Print and shaded views of the part. All mm, measured from the part's lowest x, y and z. A direction names the side the tool comes from. Round coordinates to 2 decimals unless told otherwise and drop trailing zeros. Order: outer loops, then holes, each group sorted by start corner. A loop starts at its lowest first (then second) coordinate and runs counter-clockwise, first axis right, second up. Notation, with made-up numbers: (81, 29) - (99, 29) arc R30 cw to (99, 61) - close; hole circle Ø7 at (18.5, 88.25). An arc over 180 degrees is marked (long way). Return JSON: item names as keys, results as strings. Group by question number.
Item 1: Probe probe 1 along X at (y, z) = (39.5, 5.75); probe 2 along Y at (x, z) = (40, 2.15); probe 3 along Z at (x, y) = (44, 29). List the from-to ranges inside material, lowest first.
Item 2: Saw through at A-A on x = 40. List the corners of the cut face in (y, z).
Item 3: Saw through at D-D on x = 15. List the corners of the cut face in (y, z) (1 decimal).
Item 4: Saw through at C-C on z = 5.75. List the corners of the cut face in (x, y), and give its area (3 significant figures).
Item 5: Drop flat-ended pins along their axis: pin 1 (1 mm diameter, centred on x = 48, z = 5, fed in from -Y); pin 2 (14 mm diameter, centred on x = 36, y = 32, fed in from +Z); pin 3 (5 mm diameter, centred on y = 5, z = 5, fed in from +X); pin 4 (3 mm diameter, centred on x = 10, y = 21.5, fed in from -Z). Give the stop position or say it passes through.
Item 6: Saw through at B-B on y = 42.5. List the corners of the cut face in (x, z).
Item 7: Two-plate mould, pull along X, no slides. Class the marked faces 1, 2, 3 and 4: released by +X, released by -X, zero draft, split by the parting line, or undercut.
Item 8: Tool access for the marked faces 5, 6 and 7: list every direction of +Z, -Z, +X, -X, +Y, -Y with a clear straight run to the whole face (end or side of a thin tool).
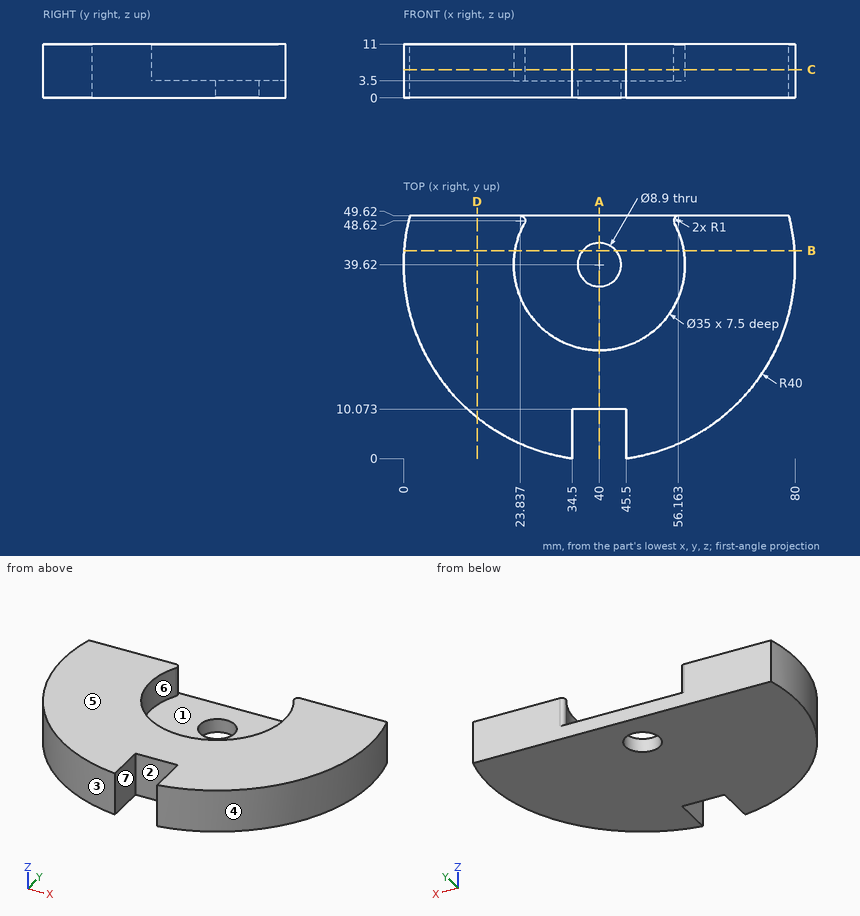
Filled in:
{
 "1": {"probe 1": "x = 0 to 22.5, 57.5 to 80", "probe 2": "y = 10.07 to 35.17, 44.07 to 49.62", "probe 3": "z = 0 to 3.5"},
 "2": {"outline": "(10.07, 0) - (35.17, 0) - (35.17, 3.5) - (22.12, 3.5) - (22.12, 11) - (10.07, 11) - close; (44.07, 0) - (49.62, 0) - (49.62, 3.5) - (44.07, 3.5) - close"},
 "3": {"outline": "(8.4, 0) - (49.6, 0) - (49.6, 11) - (8.4, 11) - close"},
 "4": {"outline": "(1.27, 49.62) arc R40 ccw to (34.5, 0) - (34.5, 10.07) - (45.5, 10.07) - (45.5, 0) arc R40 ccw to (78.73, 49.62) - (56.16, 49.62) arc R1 ccw to (55.29, 48.13) arc R17.5 cw (long way) to (24.71, 48.13) arc R1 ccw to (23.84, 49.62) - close", "area": "2,380 mm^2"},
 "5": {"pin 1": "stops at y = 0.33", "pin 2": "stops at z = 3.5", "pin 3": "stops at x = 63.84", "pin 4": "stops at z = 0"},
 "6": {"outline": "(0.1, 0) - (36.61, 0) - (36.61, 3.5) - (22.74, 3.5) - (22.74, 11) - (0.1, 11) - close; (43.39, 0) - (79.9, 0) - (79.9, 11) - (57.26, 11) - (57.26, 3.5) - (43.39, 3.5) - close"},
 "7": {"face 1": "undercut", "face 2": "undercut", "face 3": "released by -X", "face 4": "released by +X"},
 "8": {"face 5": "+Z, +X, -X, +Y, -Y", "face 6": "+Z", "face 7": "+Z, -Z, -Y"}
}
